Verification items for the finished model (mm, model axes). Round coordinates to 2 decimals unless told otherwise and drop trailing zeros. Loops run counter-clockwise (first coordinate to the right, second up) from the corner with the lowest first, then second, coordinate; pieces in that order, holes last. Notation, with made-up numbers: (35, 89.5) -> (60, 89.5) arc R27 cw to (60, 123.5) -> close; hole circle Ø4 at (72.25, -38). An arc over 180 degrees is marked (long way). Write item = value, one per line. Start each with the question number.
```python
from build123d import *

# Parameters (mm, degrees)
F0_W     = 170
F0_H     = 130
F1_DEPTH = 3
F2_W     = 10
F2_H     = 3
F2_W_2   = 3
F2_H_2   = 10
F3_DEPTH = 3.001


with BuildPart() as f1:
    # F0 (on Top) → F1 (new body)
    with BuildSketch(Plane.XY):
        Rectangle(F0_W, F0_H)
    extrude(amount=F1_DEPTH)

    # F2 (on face) → F3 (cut, through all)
    with BuildSketch(Plane.XY.offset(3)):
        with Locations((-70, -63.5)):
            Rectangle(F2_W, F2_H)
        with Locations((-50, -63.5)):
            Rectangle(F2_W, F2_H)
        with Locations((-30, -63.5)):
            Rectangle(F2_W, F2_H)
        with Locations((-10, -63.5)):
            Rectangle(F2_W, F2_H)
        with Locations((10, -63.5)):
            Rectangle(F2_W, F2_H)
        with Locations((30, -63.5)):
            Rectangle(F2_W, F2_H)
        with Locations((50, -63.5)):
            Rectangle(F2_W, F2_H)
        with Locations((70, -63.5)):
            Rectangle(F2_W, F2_H)
        with Locations((-83.5, -60)):
            Rectangle(F2_W_2, F2_H_2)
        with Locations((-83.5, -40)):
            Rectangle(F2_W_2, F2_H_2)
        with Locations((-83.5, -20)):
            Rectangle(F2_W_2, F2_H_2)
        with Locations((-83.5, 0)):
            Rectangle(F2_W_2, F2_H_2)
        with Locations((-83.5, 20)):
            Rectangle(F2_W_2, F2_H_2)
        with Locations((-83.5, 40)):
            Rectangle(F2_W_2, F2_H_2)
        with Locations((-83.5, 60)):
            Rectangle(F2_W_2, F2_H_2)
        with Locations((83.5, -60)):
            Rectangle(F2_W_2, F2_H_2)
        with Locations((83.5, -40)):
            Rectangle(F2_W_2, F2_H_2)
        with Locations((83.5, 20)):
            Rectangle(F2_W_2, F2_H_2)
        with Locations((83.5, 60)):
            Rectangle(F2_W_2, F2_H_2)
        with Locations((83.5, 0)):
            Rectangle(F2_W_2, F2_H_2)
        with Locations((83.5, -20)):
            Rectangle(F2_W_2, F2_H_2)
        with Locations((83.5, 40)):
            Rectangle(F2_W_2, F2_H_2)
        with Locations((10, 63.5)):
            Rectangle(F2_W, F2_H)
        with Locations((-70, 63.5)):
            Rectangle(F2_W, F2_H)
        with Locations((50, 63.5)):
            Rectangle(F2_W, F2_H)
        with Locations((70, 63.5)):
            Rectangle(F2_W, F2_H)
        with Locations((-30, 63.5)):
            Rectangle(F2_W, F2_H)
        with Locations((-50, 63.5)):
            Rectangle(F2_W, F2_H)
        with Locations((30, 63.5)):
            Rectangle(F2_W, F2_H)
        with Locations((-10, 63.5)):
            Rectangle(F2_W, F2_H)
    extrude(amount=-F3_DEPTH, mode=Mode.SUBTRACT)


solid = f1.part
```
(1) Section check A-A on y = -40. Enter the section's corners in (x, z), then the cut area to 3 significant figures.
(2) Section check B-B on x = -51. Enter the section's corners in (y, z).
(3) Depth check by flat-ended pin: pin 1 Ø0.9 at (x, z) = (69.5, 1) entering from -Y; pin 2 Ø0.9 at (x, z) = (69, 2) entering from +Y; pin 3 Ø0.9 at (y, z) = (63.5, 1.5) entering from -X. Enter the tip coordinate at first touch or a pass-through.
(4) Scan lines: line 1 (X direction, y = 2.5, z = 1.35); line 2 (Y direction, x = -46, z = 2.65). Record each from-to range of solid material in increasing order. Write a range as [from, to].
Computed values:
q1.outline = (-82, 0) -> (82, 0) -> (82, 3) -> (-82, 3) -> close
q1.area = 492 mm²
q2.outline = (-62, 0) -> (62, 0) -> (62, 3) -> (-62, 3) -> close
q3.pin_1 = -62
q3.pin_2 = 62
q3.pin_3 = -82
q4.line_1 = [-82, 82]
q4.line_2 = [-62, 62]
